The drawing under review shows one solid part. Ordinate dimensions are in mm from its lowest x, y, z. A direction names the side the tool comes from. Coordinates: 2 decimals unless noted, no trailing zeros. Write each loop counter-clockwise with the first axis right and the second up, starting at its lowest first coordinate (ties: lowest second). Pieces come first, ordered by that corner, then holes.
Q1. Mouldability with a two-part tool opening along Y and no side actions: class the marked faces 1, 2 and 3 as pulls with the +Y half, pulls with the -Y half, needs draft (parallel to the pull), parting line crosses it, or undercut.
Q2. Machinability: for the marked faces 4, 5, 6 and 7, which of the approach directions +Z, -Z, +X, -X, +Y, -Y give a long, thin tool a straight path to every point of the face, cutting with its end or side? Answer none if there is none.
Q3. Take a section at B-B (y = 92). Give the boundary of the cut face in (x, z).
Q4. Take a section at C-C (z = 82). Give the boundary of the cut face in (x, y).
Q5. Take a section at A-A (y = 10). Give the boundary of the cut face in (x, z).
Q6. Take a section at D-D (y = 57). Give the boundary of the cut face in (x, z).
Q7. For probe 1 along Y at (x, z) = (91.5, 64); probe 2 along Z at (x, y) = (18.5, 5); probe 3 along X at (y, z) = (14, 20), list the stretches that pass through material, from the lowest coordinate up.
Q8. Insertion check: pin 1 (7.5 mm diameter, centred on y = 35.5, z = 66.5, fed in from -X); pin 2 (1.5 mm diameter, centred on x = 53.5, y = 33.5, fed in from -Z); pin 3 (8 mm diameter, centred on x = 88, z = 68, fed in from +Y). Each pin has a flat end and moves straight along its axis. Give the tip position at first contact, or say it passes through.
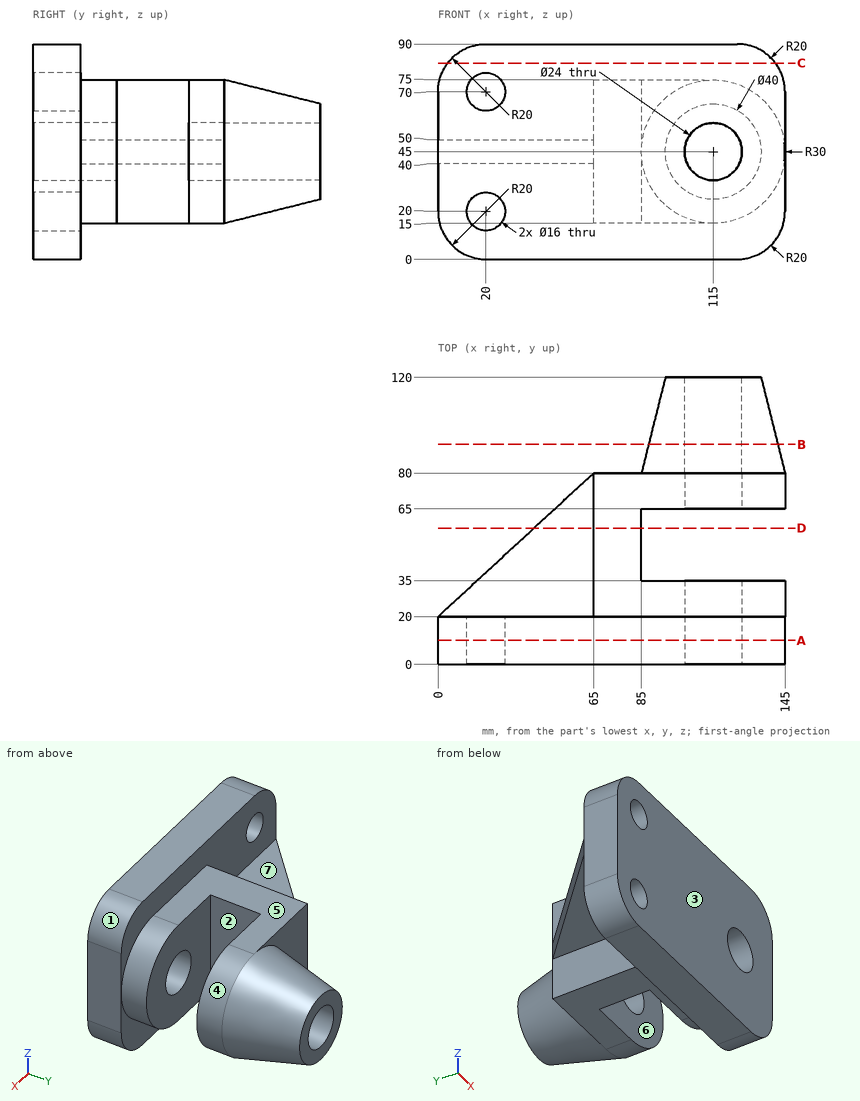
Response:
1. face 1: needs draft
1. face 2: undercut
1. face 3: pulls with the -Y half
2. face 4: +X, +Y
2. face 5: +Z, +X, -X, +Y
2. face 6: +Z, -Z, +X
2. face 7: +Z, -X, +Y
3. outline: circle Ø54 at (115, 45); hole circle Ø24 at (115, 45)
4. outline: (4, 0) - (141, 0) - (141, 20) - (4, 20) - close
5. outline: (0, 20) arc R20 ccw to (20, 0) - (125, 0) arc R20 ccw to (145, 20) - (145, 70) arc R20 ccw to (125, 90) - (20, 90) arc R20 ccw to (0, 70) - close; hole circle Ø16 at (20, 20); hole circle Ø16 at (20, 70); hole circle Ø24 at (115, 45)
6. outline: (40.08, 40) - (65, 40) - (65, 15) - (85, 15) - (85, 75) - (65, 75) - (65, 50) - (40.08, 50) - close
7. probe 1: y = 0 to 35, 65 to 80
7. probe 2: z = 0.06 to 12.14, 27.86 to 62.14, 77.86 to 89.94
7. probe 3: x = 0 to 12, 28 to 145
8. pin 1: stops at x = 65
8. pin 2: stops at z = 40
8. pin 3: stops at y = 80
